Source: CAD feature listing. Evaluate the final solid. Frame: model axes, mm. Face numbers are marked on the shaded views. Coordinates: 2 decimals unless noted, no trailing zeros. Loops run counter-clockwise (first coordinate to the right, second up) from the corner with the lowest first, then second, coordinate; pieces in that order, holes last. Notation, with made-up numbers: (-34.5, 78.5) - (13.5, 78.5) arc R22 cw to (13.5, 108.5) - close; hole circle Ø9 at (89, 58.5). An arc over 180 degrees is marked (long way). Use CSV: the item, a comma, the result in double quotes. Start each with the question number.
```python
from build123d import *

# Parameters (mm, degrees)
F0_W     = 15
F0_H     = 15.8
F0_R     = 3
F0_R_2   = 1.6
F1_DEPTH = 11
F2_DEPTH = 5
F3_R     = 2


with BuildPart() as f1:
    # F0 (on Top) → F1 (new body)
    with BuildSketch(Plane.XY):
        Rectangle(F0_W, F0_H)
        Circle(F0_R, mode=Mode.SUBTRACT)
        Circle(F0_R)
        Circle(F0_R_2, mode=Mode.SUBTRACT)
    extrude(amount=F1_DEPTH)

    # F0 (on Top) → F2 (cut)
    with BuildSketch(Plane.XY):
        Circle(F0_R)
        Circle(F0_R_2, mode=Mode.SUBTRACT)
    extrude(amount=F2_DEPTH, mode=Mode.SUBTRACT)

    # F3
    f3_edges = [f1.edges().sort_by_distance(p)[0] for p in [
        (-7.5, 7.9, 5.5),
        (-7.5, -7.9, 5.5),
        (7.5, -7.9, 5.5),
        (7.5, 7.9, 5.5),
    ]]
    fillet(f3_edges, radius=F3_R)


solid = f1.part
```
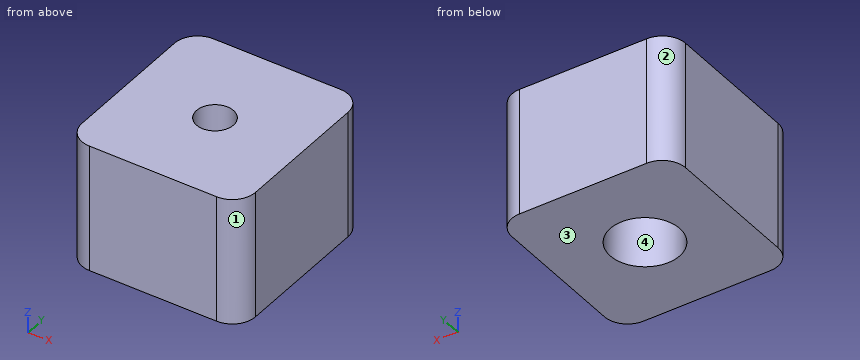
(1) Section B-B on z = 7.5. Output: boundary loops of the cut face in (x, y), plus the area to 3 significant figures.
(2) Section C-C on x = 0. Output: boundary loops of the cut face in (y, z).
(3) Pin query (flat end, axial travel): pin 1 Ø1.9 at (x, y) = (0, 0) entering from -Z; pin 2 Ø8 at (x, y) = (0, 0) entering from +Z. Return the tip coordinate at first contact, or that it passes through.
(4) Section A-A on y = 0. Output: boundary loops of the cut face in (x, z).
(5) Draft query along Y for the marked faces 1, 2, 3 and 4. Return one class per face: released by +Y, released by -Y, zero draft, split by the parting line, or undercut.
(6) Ray query, line 1 (Y direction, x = 0, z = 2.05); line 2 (Y direction, x = 0, z = 9.8); line 3 (Z direction, x = -1.75, y = -1.25). Return the intervals inside material, ascending. Write a range as [from, to].
(7) Section D-D on x = 2. Output: boundary loops of the cut face in (y, z).
Solution:
1,outline,"(-7.5, -5.9) arc R2 ccw to (-5.5, -7.9) - (5.5, -7.9) arc R2 ccw to (7.5, -5.9) - (7.5, 5.9) arc R2 ccw to (5.5, 7.9) - (-5.5, 7.9) arc R2 ccw to (-7.5, 5.9) - close; hole circle Ø3.2 at (0, 0)"
1,area,"226 mm²"
2,outline,"(-7.9, 0) - (-3, 0) - (-3, 5) - (-1.6, 5) - (-1.6, 11) - (-7.9, 11) - close; (1.6, 5) - (3, 5) - (3, 0) - (7.9, 0) - (7.9, 11) - (1.6, 11) - close"
3,pin 1,"passes through"
3,pin 2,"stops at z = 11"
4,outline,"(-7.5, 0) - (-3, 0) - (-3, 5) - (-1.6, 5) - (-1.6, 11) - (-7.5, 11) - close; (1.6, 5) - (3, 5) - (3, 0) - (7.5, 0) - (7.5, 11) - (1.6, 11) - close"
5,face 1,"released by -Y"
5,face 2,"released by +Y"
5,face 3,"zero draft"
5,face 4,"undercut"
6,line 1,"y = [-7.9, -3], [3, 7.9]"
6,line 2,"y = [-7.9, -1.6], [1.6, 7.9]"
6,line 3,"z = [5, 11]"
7,outline,"(-7.9, 0) - (-2.24, 0) - (-2.24, 5) - (2.24, 5) - (2.24, 0) - (7.9, 0) - (7.9, 11) - (-7.9, 11) - close"
